Could you check a few things on this model? Use its own coordinates, in mm. A direction names the side the tool comes from. Coordinates: 2 decimals unless noted, no trailing zeros. Order: outer loops, then holes, each group sorted by start corner. A loop starts at its lowest first (then second) coordinate and runs counter-clockwise, first axis right, second up. Notation, with made-up numbers: (16.5, 14) - (52.5, 14) arc R32 ccw to (52.5, 48) - close; hole circle Ø11 at (54.25, 4). An arc over 180 degrees is marked (long way). Answer as CSV lines item,"result". Start each with the question number.
1. I want a section at C-C, the plane y = -5.25. List the corners of the cut face in (x, z) for me.
2. I need wall thicknesses on probe 1 along X at (y, z) = (8.75, 1); probe 2 along Z at (x, y) = (-8.75, -3.5); probe 3 along Z at (x, y) = (0.5, 8). Which ranges of each line are inside material? Lowest first, please.
3. I want a section at A-A, the plane x = 0. List the corners of the cut face in (y, z) for me, and give its area (3 significant figures).
4. For faces 5 (the face through (1.071, 8.432, 0.056)), 6 (the face through (6, 0, -7)), 7 (the face through (-7.5, -4.4, -4)), 8 (the face through (-8.484, -0.528, 0.056)), 9 (the face through (-2.6, 0, -2)), which set-ups out of +Z, -Z, +X, -X, +Y, -Y let a thin tool reach every point of the face, with its end or its side?
5. Thinking about a two-plate mould opening in X: for faces 1 (the face through (-2.17, -9.76, -4.51)), 2 (the face through (0, -7, -5)), 3 (the face through (2.6, 0, -2)), 4 (the face through (0, -2.6, -2)), which applies, released by +X, released by -X, zero draft, split by the parting line, or undercut?
6. I want a section at B-B, the plane z = -5.75. List the corners of the cut face in (x, y) for me, and give its area (3 significant figures).
7. For pin 1 (10 mm diameter, centred on x = 6, y = -3.5, fed in from -Z); pin 2 (0.6 mm diameter, centred on x = 0, z = 0, fed in from +Y); pin 3 (2 mm diameter, centred on x = 7, z = -2.5, fed in from -Y); pin 4 (1.6 mm diameter, centred on x = -1, z = 1, fed in from -Y), each with a flat end and sliding along its axis, tell me the tip position at first contact or that it passes through.
from build123d import *

# Parameters (mm, degrees)
BOSS_EXTRUDE1_DEPTH = 5
SKETCH2_R           = 10
BOSS_EXTRUDE2_DEPTH = 1
SKETCH4_R           = 6
BOSS_EXTRUDE3_DEPTH = 5
CUT_EXTRUDE1_REACH  = 17
SKETCH5_W           = 5.2
SKETCH5_H           = 5.2


with BuildPart() as part:
    # Sketch1 → Boss-Extrude1 (new body, symmetric)
    with BuildSketch(Plane.XY):
        with BuildLine():
            Line((-0.4, 9.191300234), (-0.660980834, 8.474261286))
            ThreePointArc((-0.660980834, 8.474261286), (-1.065332485, 8.432974961), (-1.467248177, 8.372406033))
            Line((-1.467248177, 8.372406033), (-1.898350154, 9.002014591))
            Line((-1.898350154, 9.002014591), (-2.673216683, 8.803062681))
            Line((-2.673216683, 8.803062681), (-2.747677989, 8.043647535))
            ThreePointArc((-2.747677989, 8.043647535), (-3.129058698, 7.90310013), (-3.503284589, 7.744481718))
            Line((-3.503284589, 7.744481718), (-4.077419986, 8.247099263))
            Line((-4.077419986, 8.247099263), (-4.77846533, 7.861696324))
            Line((-4.77846533, 7.861696324), (-4.66172843, 7.107621828))
            ThreePointArc((-4.66172843, 7.107621828), (-4.996174644, 6.876644452), (-5.319196746, 6.629943135))
            Line((-5.319196746, 6.629943135), (-6.000290524, 6.973988359))
            Line((-6.000290524, 6.973988359), (-6.583465426, 6.426350674))
            Line((-6.583465426, 6.426350674), (-6.282865329, 5.724998101))
            ThreePointArc((-6.282865329, 5.724998101), (-6.549362564, 5.418103913), (-6.80088421, 5.098820841))
            Line((-6.80088421, 5.098820841), (-7.546140742, 5.262676117))
            Line((-7.546140742, 5.262676117), (-7.974802178, 4.587213776))
            Line((-7.974802178, 4.587213776), (-7.509226693, 3.982651688))
            ThreePointArc((-7.509226693, 3.982651688), (-7.691029946, 3.619123978), (-7.855247106, 3.247320882))
            Line((-7.855247106, 3.247320882), (-8.617839183, 3.220690579))
            Line((-8.617839183, 3.220690579), (-8.865052779, 2.459845366))
            Line((-8.865052779, 2.459845366), (-8.263755727, 1.990060623))
            ThreePointArc((-8.263755727, 1.990060623), (-8.349441631, 1.592741174), (-8.416035937, 1.191779808))
            Line((-8.416035937, 1.191779808), (-9.148047095, 0.976337208))
            Line((-9.148047095, 0.976337208), (-9.198279511, 0.177915826))
            Line((-9.198279511, 0.177915826), (-8.499042597, -0.127573271))
            ThreePointArc((-8.499042597, -0.127573271), (-8.483227192, -0.533719416), (-8.448014278, -0.938645173))
            Line((-8.448014278, -0.938645173), (-9.103449564, -1.32936302))
            Line((-9.103449564, -1.32936302), (-8.953544512, -2.115192821))
            Line((-8.953544512, -2.115192821), (-8.200303363, -2.237191266))
            ThreePointArc((-8.200303363, -2.237191266), (-8.083980389, -2.626644452), (-7.949172812, -3.010091627))
            Line((-7.949172812, -3.010091627), (-8.486848816, -3.551534481))
            Line((-8.486848816, -3.551534481), (-8.146225383, -4.275396123))
            Line((-8.146225383, -4.275396123), (-7.38630891, -4.206238307))
            ThreePointArc((-7.38630891, -4.206238307), (-7.176787367, -4.554527757), (-6.950855584, -4.892402953))
            Line((-6.950855584, -4.892402953), (-7.336988145, -5.550549969))
            Line((-7.336988145, -5.550549969), (-6.827048953, -6.166960564))
            Line((-6.827048953, -6.166960564), (-6.108205503, -5.910991925))
            ThreePointArc((-6.108205503, -5.910991925), (-5.8186504, -6.196233333), (-5.515790536, -6.467306608))
            Line((-5.515790536, -6.467306608), (-5.726117525, -7.200803989))
            Line((-5.726117525, -7.200803989), (-5.078903929, -7.671032191))
            Line((-5.078903929, -7.671032191), (-4.44630108, -7.244336181))
            ThreePointArc((-4.44630108, -7.244336181), (-4.09490623, -7.44860678), (-3.734148082, -7.635845605))
            Line((-3.734148082, -7.635845605), (-3.755453882, -8.398605012))
            Line((-3.755453882, -8.398605012), (-3.011632693, -8.693104654))
            Line((-3.011632693, -8.693104654), (-2.505019208, -8.122492153))
            ThreePointArc((-2.505019208, -8.122492153), (-2.113864041, -8.23295687), (-1.717875372, -8.324596339))
            Line((-1.717875372, -8.324596339), (-1.54882126, -9.068690793))
            Line((-1.54882126, -9.068690793), (-0.755129499, -9.16895738))
            Line((-0.755129499, -9.16895738), (-0.406337766, -8.49028207))
            ThreePointArc((-0.406337766, -8.49028207), (0, -8.5), (0.406337766, -8.49028207))
            Line((0.406337766, -8.49028207), (0.755129499, -9.16895738))
            Line((0.755129499, -9.16895738), (1.54882126, -9.068690793))
            Line((1.54882126, -9.068690793), (1.717875372, -8.324596339))
            ThreePointArc((1.717875372, -8.324596339), (2.113864041, -8.23295687), (2.505019208, -8.122492153))
            Line((2.505019208, -8.122492153), (3.011632693, -8.693104654))
            Line((3.011632693, -8.693104654), (3.755453882, -8.398605012))
            Line((3.755453882, -8.398605012), (3.734148082, -7.635845605))
            ThreePointArc((3.734148082, -7.635845605), (4.09490623, -7.44860678), (4.44630108, -7.244336181))
            Line((4.44630108, -7.244336181), (5.078903929, -7.671032191))
            Line((5.078903929, -7.671032191), (5.726117525, -7.200803989))
            Line((5.726117525, -7.200803989), (5.515790536, -6.467306608))
            ThreePointArc((5.515790536, -6.467306608), (5.8186504, -6.196233333), (6.108205503, -5.910991925))
            Line((6.108205503, -5.910991925), (6.827048953, -6.166960564))
            Line((6.827048953, -6.166960564), (7.336988145, -5.550549969))
            Line((7.336988145, -5.550549969), (6.950855584, -4.892402953))
            ThreePointArc((6.950855584, -4.892402953), (7.176787367, -4.554527757), (7.38630891, -4.206238307))
            Line((7.38630891, -4.206238307), (8.146225383, -4.275396123))
            Line((8.146225383, -4.275396123), (8.486848816, -3.551534481))
            Line((8.486848816, -3.551534481), (7.949172812, -3.010091627))
            ThreePointArc((7.949172812, -3.010091627), (8.083980389, -2.626644452), (8.200303363, -2.237191266))
            Line((8.200303363, -2.237191266), (8.953544512, -2.115192821))
            Line((8.953544512, -2.115192821), (9.103449564, -1.32936302))
            Line((9.103449564, -1.32936302), (8.448014278, -0.938645173))
            ThreePointArc((8.448014278, -0.938645173), (8.483227192, -0.533719416), (8.499042597, -0.127573271))
            Line((8.499042597, -0.127573271), (9.198279511, 0.177915826))
            Line((9.198279511, 0.177915826), (9.148047095, 0.976337208))
            Line((9.148047095, 0.976337208), (8.416035937, 1.191779808))
            ThreePointArc((8.416035937, 1.191779808), (8.349441631, 1.592741174), (8.263755727, 1.990060623))
            Line((8.263755727, 1.990060623), (8.865052779, 2.459845366))
            Line((8.865052779, 2.459845366), (8.617839183, 3.220690579))
            Line((8.617839183, 3.220690579), (7.855247106, 3.247320882))
            ThreePointArc((7.855247106, 3.247320882), (7.691029946, 3.619123978), (7.509226693, 3.982651688))
            Line((7.509226693, 3.982651688), (7.974802178, 4.587213776))
            Line((7.974802178, 4.587213776), (7.546140742, 5.262676117))
            Line((7.546140742, 5.262676117), (6.80088421, 5.098820841))
            ThreePointArc((6.80088421, 5.098820841), (6.549362564, 5.418103913), (6.282865329, 5.724998101))
            Line((6.282865329, 5.724998101), (6.583465426, 6.426350674))
            Line((6.583465426, 6.426350674), (6.000290524, 6.973988359))
            Line((6.000290524, 6.973988359), (5.319196746, 6.629943135))
            ThreePointArc((5.319196746, 6.629943135), (4.996174644, 6.876644452), (4.66172843, 7.107621828))
            Line((4.66172843, 7.107621828), (4.77846533, 7.861696324))
            Line((4.77846533, 7.861696324), (4.077419986, 8.247099263))
            Line((4.077419986, 8.247099263), (3.503284589, 7.744481718))
            ThreePointArc((3.503284589, 7.744481718), (3.129058698, 7.90310013), (2.747677989, 8.043647535))
            Line((2.747677989, 8.043647535), (2.673216683, 8.803062681))
            Line((2.673216683, 8.803062681), (1.898350154, 9.002014591))
            Line((1.898350154, 9.002014591), (1.467248177, 8.372406033))
            ThreePointArc((1.467248177, 8.372406033), (1.065332485, 8.432974961), (0.660980834, 8.474261286))
            Line((0.660980834, 8.474261286), (0.4, 9.191300234))
            Line((0.4, 9.191300234), (-0.4, 9.191300234))
        make_face()
    extrude(amount=BOSS_EXTRUDE1_DEPTH, both=True)

    # Sketch2 → Boss-Extrude2 (add)
    with BuildSketch(Plane.XY.offset(5)):
        Circle(SKETCH2_R)
    boss_extrude2 = extrude(amount=-BOSS_EXTRUDE2_DEPTH)

    # Mirror1: Boss-Extrude2 across plane
    add(boss_extrude2.mirror(Plane.XY))

    # Sketch4 → Boss-Extrude3 (add)
    with BuildSketch(Plane(origin=(0, 0, -5), x_dir=(-1, 0, 0), z_dir=(0, 0, -1))):
        Circle(SKETCH4_R)
    extrude(amount=BOSS_EXTRUDE3_DEPTH)

    # Sketch5 → Cut-Extrude1 (cut, up to next)
    with BuildSketch(Plane.XY.offset(5), mode=Mode.PRIVATE) as cut_extrude1_sk1:
        Rectangle(SKETCH5_W, SKETCH5_H)
    cut_extrude1_tool1 = extrude(cut_extrude1_sk1.sketch, amount=-CUT_EXTRUDE1_REACH, mode=Mode.PRIVATE) & part.part
    add(cut_extrude1_tool1.solids().sort_by_distance((0, 0, 5))[0], mode=Mode.SUBTRACT)


solid = part.part
Solved:
1,outline,"(-8.51, -5) - (-2.9, -5) - (-2.9, -10) - (2.9, -10) - (2.9, -5) - (8.51, -5) - (8.51, -4) - (7.16, -4) - (7.16, 4) - (8.51, 4) - (8.51, 5) - (-8.51, 5) - (-8.51, 4) - (-7.16, 4) - (-7.16, -4) - (-8.51, -4) - close"
2,probe 1,"x = -2.68 to -1.73, -0.56 to 0.56, 1.73 to 2.68"
2,probe 2,"z = -5 to -4, 4 to 5"
2,probe 3,"z = -5 to 5"
3,outline,"(-10, -5) - (-6, -5) - (-6, -10) - (-2.6, -10) - (-2.6, 5) - (-10, 5) - (-10, 4) - (-8.5, 4) - (-8.5, -4) - (-10, -4) - close; (2.6, -10) - (6, -10) - (6, -5) - (10, -5) - (10, -4) - (9.19, -4) - (9.19, 4) - (10, 4) - (10, 5) - (2.6, 5) - close"
3,area,"164 mm2"
4,face 5,"+Y"
4,face 6,"-Z"
4,face 7,"none"
4,face 8,"-X"
4,face 9,"+Z, -Z"
5,face 1,"split by the parting line"
5,face 2,"zero draft"
5,face 3,"undercut"
5,face 4,"undercut"
6,outline,"circle Ø12 at (0, 0); hole (-2.6, -2.6) - (2.6, -2.6) - (2.6, 2.6) - (-2.6, 2.6) - close"
6,area,"86.1 mm2"
7,pin 1,"stops at z = -10"
7,pin 2,"stops at y = 9.19"
7,pin 3,"stops at y = -6.17"
7,pin 4,"stops at y = -9.17"
